```python
from build123d import *

# Parameters (mm, degrees)
ESQUISSE1_W             = 10
ESQUISSE1_H             = 150
BOSS_EXTRU_1_DEPTH      = 5
CONG_1_RADIUS           = 5
CONG_1_LENGTH           = 5
CONG_2_RADIUS           = 5
CONG_2_LENGTH           = 5
ESQUISSE2_R             = 2.5
ESQUISSE2_R_2           = 1.5
ENL_V_MAT_EXTRU_1_DEPTH = 76.332595867
ESQUISSE3_R             = 2.5
BOSS_EXTRU_2_DEPTH      = 2.5


with BuildPart() as part:
    # Esquisse1 → Boss.-Extru.1 (new body)
    with BuildSketch(Plane.XY):
        Rectangle(ESQUISSE1_W, ESQUISSE1_H)
    extrude(amount=BOSS_EXTRU_1_DEPTH)

    # Congé1: full round fillet: the end face becomes a half cylinder, R = half its width
    cong_1_face = Plane((0, 75, 2.5), x_dir=(0, 0, 1), z_dir=(0, 1, 0))  # on the end face: x along it, z out of the body
    cong_1_slab = cong_1_face.offset(-CONG_1_RADIUS / 2) * Box(CONG_1_LENGTH, 2 * CONG_1_RADIUS, CONG_1_RADIUS, mode=Mode.PRIVATE)  # the body's end, R deep
    cong_1_round = Plane((0, 70, 2.5), x_dir=(0, 1, 0), z_dir=(0, 0, 1)) * Cylinder(CONG_1_RADIUS, CONG_1_LENGTH, mode=Mode.PRIVATE)  # its axis R under the face
    add(cong_1_slab - cong_1_round, mode=Mode.SUBTRACT)

    # Congé2: full round fillet: the end face becomes a half cylinder, R = half its width
    cong_2_face = Plane((0, -75, 2.5), x_dir=(0, 0, 1), z_dir=(0, -1, 0))  # on the end face: x along it, z out of the body
    cong_2_slab = cong_2_face.offset(-CONG_2_RADIUS / 2) * Box(CONG_2_LENGTH, 2 * CONG_2_RADIUS, CONG_2_RADIUS, mode=Mode.PRIVATE)  # the body's end, R deep
    cong_2_round = Plane((0, -70, 2.5), x_dir=(0, -1, 0), z_dir=(0, 0, 1)) * Cylinder(CONG_2_RADIUS, CONG_2_LENGTH, mode=Mode.PRIVATE)  # its axis R under the face
    add(cong_2_slab - cong_2_round, mode=Mode.SUBTRACT)

    # Esquisse2 → Enlèv. mat.-Extru.1 (cut, through all)
    with BuildSketch(Plane.XY.offset(5)):
        with Locations((0, 70)):
            Circle(ESQUISSE2_R)
        with Locations((0, -70)):
            Circle(ESQUISSE2_R_2)
    extrude(amount=-ENL_V_MAT_EXTRU_1_DEPTH, mode=Mode.SUBTRACT)

    # Esquisse3 → Boss.-Extru.2 (add)
    with BuildSketch(Plane.XY.offset(5)):
        with Locations((0, 70)):
            Circle(ESQUISSE3_R)
    extrude(amount=-BOSS_EXTRU_2_DEPTH)


solid = part.part
```
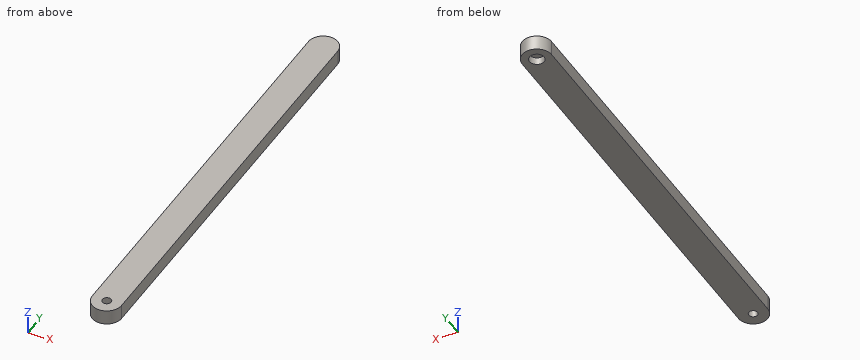
Can you work these out from the model? Positions are in its coordinate system, mm. Round coordinates to 2 decimals unless told otherwise and drop trailing zeros. Loops run counter-clockwise (first coordinate to the right, second up) from the corner with the lowest first, then second, coordinate; pieces in that order, holes last. Notation, with made-up numbers: M 4,46 L 30,46 A13 ccw 30,57 Z; hole C -2.5,55 d5. An arc over 180 degrees is marked long. Answer in a Markdown table with one row per item.
1. If we section it at B-B, the plane z = 3.5: Please give me the cut outline in (x, y), plus the area to 3 significant figures.
Established:
| item | result |
|---|---|
| outline | M -5,-70 A5 ccw 5,-70 L 5,70 A5 ccw -5,70 Z; hole C 0,-70 d3 |
| area | 1,470 mm² |
2. Please list where these lines run through material, in increasing order: line 1 (Y direction, x = 0, z = 3.65); line 2 (Y direction, x = 0, z = 0.75); line 3 (X direction, y = -70, z = 2.3). Write a range as from..to.
Established:
| item | result |
|---|---|
| line 1 | -75..-71.5, -68.5..75 |
| line 2 | -75..-71.5, -68.5..67.5, 72.5..75 |
| line 3 | -5..-1.5, 1.5..5 |
3. I'm going to push a flat-ended pin straight in: pin 1 Ø1.5 at (x, z) = (-4, 4.5) entering from -Y. Where does the tip first touch, or does it pass through?
Established:
| item | result |
|---|---|
| pin 1 | y = -73.8 |
4. If we section it at A-A, the plane x = 0: Please give me the cut outline in (y, z), plus the area to 4 significant figures.
Established:
| item | result |
|---|---|
| outline | M -75,0 L -71.5,0 L -71.5,5 L -75,5 Z; M -68.5,0 L 67.5,0 L 67.5,2.5 L 72.5,2.5 L 72.5,0 L 75,0 L 75,5 L -68.5,5 Z |
| area | 722.5 mm² |
